```python
from build123d import *

# Parameters (mm, degrees)
CROQUIS1_R                   = 6
SALIENTE_EXTRUIR1_DEPTH      = 16.5
CROQUIS2_R                   = 4.2
CORTAR_EXTRUIR1_DEPTH        = 14.5
CROQUIS3_R                   = 2.6
SALIENTE_EXTRUIR2_DEPTH      = 6
CORTAR_EXTRUIR4_START        = -6
CORTAR_EXTRUIR4_DEPTH        = 6
CORTAR_EXTRUIR5_START        = -6
CORTAR_EXTRUIR5_DEPTH        = 6
SALIENTE_EXTRUIR3_DEPTH      = 6
SALIENTE_EXTRUIR3_DEPTH_BACK = 12
CROQUIS13_R                  = 7
CROQUIS13_R_2                = 4.7
CORTAR_EXTRUIR9_REACH        = 26.581
CORTAR_EXTRUIR9_END_RADIUS   = 7
CROQUIS14_R                  = 1.4


with BuildPart() as part:
    # Croquis1 → Saliente-Extruir1 (new body)
    with BuildSketch(Plane(origin=(0, 0, 0), x_dir=(1, 0, 0), z_dir=(0, 1, 0))):
        with Locations(Location((0, 0, 0), (0, 0, 270))):
            Circle(CROQUIS1_R)
    extrude(amount=SALIENTE_EXTRUIR1_DEPTH)

    # Croquis2 → Cortar-Extruir1 (cut)
    with BuildSketch(Plane.XZ):
        with Locations(Location((0, 0, 0), (0, 0, 270))):
            Circle(CROQUIS2_R)
    extrude(amount=-CORTAR_EXTRUIR1_DEPTH, mode=Mode.SUBTRACT)

    # Croquis3 → Saliente-Extruir2 (add)
    with BuildSketch(Plane(origin=(0, 16.5, 0), x_dir=(1, 0, 0), z_dir=(0, 1, 0))):
        with Locations(Location((0, 0, 0), (0, 0, 270))):
            Circle(CROQUIS3_R)
    extrude(amount=SALIENTE_EXTRUIR2_DEPTH)

    # Croquis7 → Cortar-Extruir4 (cut)
    with BuildSketch(Plane(origin=(0, 22.5, 0), x_dir=(1, 0, 0), z_dir=(0, 1, 0)).offset(CORTAR_EXTRUIR4_START)):
        with BuildLine():
            Line((-1.774823935, -1.9), (1.774823935, -1.9))
            ThreePointArc((1.774823935, -1.9), (0, -2.6), (-1.774823935, -1.9))
        make_face()
        with BuildLine():
            Line((-1.774823935, 1.9), (1.774823935, 1.9))
            ThreePointArc((1.774823935, 1.9), (0, 2.6), (-1.774823935, 1.9))
        make_face()
    extrude(amount=CORTAR_EXTRUIR4_DEPTH, mode=Mode.SUBTRACT)

    # Croquis10 → Cortar-Extruir5 (cut)
    with BuildSketch(Plane(origin=(0, 22.5, 0), x_dir=(1, 0, 0), z_dir=(0, 1, 0)).offset(CORTAR_EXTRUIR5_START)):
        with BuildLine():
            Line((-1.8, 0.7), (-2.503996805, 0.7))
            ThreePointArc((-2.503996805, 0.7), (-2.6, 0), (-2.503996805, -0.7))
            Line((-2.503996805, -0.7), (-1.8, -0.7))
            Line((-1.8, -0.7), (-1.8, 0.7))
        make_face()
        with BuildLine():
            Line((2.503996805, 0.7), (1.8, 0.7))
            Line((1.8, 0.7), (1.8, -0.7))
            Line((1.8, -0.7), (2.503996805, -0.7))
            ThreePointArc((2.503996805, -0.7), (2.6, 0), (2.503996805, 0.7))
        make_face()
    extrude(amount=CORTAR_EXTRUIR5_DEPTH, mode=Mode.SUBTRACT)

    # Croquis13 → Saliente-Extruir3 (add, two sides: drawn at the far end of the back side and taken through both)
    with BuildSketch(Plane(origin=(0, 16.5, 0), x_dir=(1, 0, 0), z_dir=(0, 1, 0)).offset(-SALIENTE_EXTRUIR3_DEPTH_BACK)):
        with Locations(Location((0, 0, 0), (0, 0, 270))):
            Circle(CROQUIS13_R)
        with Locations(Location((0, 0, 0), (0, 0, 270))):
            Circle(CROQUIS13_R_2, mode=Mode.SUBTRACT)
    extrude(amount=SALIENTE_EXTRUIR3_DEPTH + SALIENTE_EXTRUIR3_DEPTH_BACK)

    # Cortar-Extruir9: up to this cylinder (the profile starts inside it)
    cortar_extruir9_end = Plane(origin=(0, 10, 0), z_dir=(0, 1, 0)) * Cylinder(CORTAR_EXTRUIR9_END_RADIUS, 68.162, mode=Mode.PRIVATE)
    # Croquis14 → Cortar-Extruir9 (cut, up to the surface)
    with BuildSketch(Plane.XY, mode=Mode.PRIVATE) as cortar_extruir9_sk1:
        with Locations((0, 10)):
            Circle(CROQUIS14_R)
    cortar_extruir9_tool1 = extrude(cortar_extruir9_sk1.sketch, amount=-CORTAR_EXTRUIR9_REACH, mode=Mode.PRIVATE) & cortar_extruir9_end
    add(cortar_extruir9_tool1.solids().sort_by_distance((0, 10, 0))[0], mode=Mode.SUBTRACT)


solid = part.part
```
Verification items for the finished model (mm, model axes). A direction names the side the tool comes from. Give positions to 0.01 mm unless a question says otherwise; leave off trailing zeros. Order: outer loops, then holes, each group sorted by start corner. A loop starts at its lowest first (then second) coordinate and runs counter-clockwise, first axis right, second up. Notation, with made-up numbers: (0.5, 59) -> (40.5, 59) arc R18 ccw to (40.5, 63) -> close; hole circle Ø5 at (49, -33.75). An arc over 180 degrees is marked (long way). Use a Markdown table: item, result.
1) Section check C-C, the plane z = 0. Record the boundary of the cut face in (x, y).
Results:
| item | result |
|---|---|
| outline | (-7, 4.5) -> (-6, 4.5) -> (-6, 0) -> (-4.2, 0) -> (-4.2, 14.5) -> (4.2, 14.5) -> (4.2, 0) -> (6, 0) -> (6, 4.5) -> (7, 4.5) -> (7, 22.5) -> (4.7, 22.5) -> (4.7, 16.5) -> (1.8, 16.5) -> (1.8, 22.5) -> (-1.8, 22.5) -> (-1.8, 16.5) -> (-4.7, 16.5) -> (-4.7, 22.5) -> (-7, 22.5) -> close |
2) Mould release check, pull along X, two halves, no side actions. Record for faces 1 (the cylindrical face through (1.802, 2.218, 5.723)), 2 (the flat face through (-5, 22.5, 1)), 3 (the flat face through (-2, 16.5, 0)): pulls with the +X half, pulls with the -X half, needs draft (parallel to the pull), parting line crosses it, or undercut.
Results:
| item | result |
|---|---|
| face 1 | parting line crosses it |
| face 2 | needs draft |
| face 3 | undercut |
3) Section check B-B, the plane z = -5.5. Record the boundary of the cut face in (x, y), then the cut area to 3 significant figures.
Results:
| item | result |
|---|---|
| outline | (-4.33, 4.5) -> (-2.4, 4.5) -> (-2.4, 0) -> (2.4, 0) -> (2.4, 4.5) -> (4.33, 4.5) -> (4.33, 22.5) -> (-4.33, 22.5) -> close; hole circle Ø2.8 at (0, 10) |
| area | 171 mm² |
4) Section check D-D, the plane y = 10. Record the boundary of the cut face in (x, z), then the cut area to 3 significant figures.
Results:
| item | result |
|---|---|
| outline | (-1.4, -6.86) -> (-1.4, -3.96) arc R4.2 cw (long way) to (1.4, -3.96) -> (1.4, -6.86) arc R7 ccw (long way) to start |
| area | 90.6 mm² |
5) Tool access check on faces 4 (the flat face through (0, 22.5, 0)), 5 (the cylindrical face through (-1.4, 10.06, -5.46)), 6 (the cylindrical face through (-2.23, 19.46, 1.34)), 7 (the flat face through (0, 14.5, 0)). Record the directions out of +Z, -Z, +X, -X, +Y, -Y that give a thin tool (end or side, any length) a straight path to the whole face; none if there is none.
Results:
| item | result |
|---|---|
| face 4 | +Z, -Z, +X, -X, +Y |
| face 5 | -Z |
| face 6 | +Y |
| face 7 | -Y |
6) Material ranges on probe 1 along X at (y, z) = (19.2, 0); probe 2 along Z at (x, y) = (0, 18.3); probe 3 along X at (y, z) = (5.5, 0), recorded low to high.
Results:
| item | result |
|---|---|
| probe 1 | -7 to -4.7, -1.8 to 1.8, 4.7 to 7 |
| probe 2 | -7 to -4.7, -1.9 to 1.9, 4.7 to 7 |
| probe 3 | -7 to -4.2, 4.2 to 7 |
7) Section check A-A, the plane x = 0. Record the boundary of the cut face in (y, z), then the cut area to 3 significant figures.
Results:
| item | result |
|---|---|
| outline | (0, -6) -> (4.5, -6) -> (4.5, -7) -> (8.6, -7) -> (8.6, -4.2) -> (0, -4.2) -> close; (0, 4.2) -> (14.5, 4.2) -> (14.5, -4.2) -> (11.4, -4.2) -> (11.4, -7) -> (22.5, -7) -> (22.5, -4.7) -> (16.5, -4.7) -> (16.5, -1.9) -> (22.5, -1.9) -> (22.5, 1.9) -> (16.5, 1.9) -> (16.5, 4.7) -> (22.5, 4.7) -> (22.5, 7) -> (4.5, 7) -> (4.5, 6) -> (0, 6) -> close |
| area | 143 mm² |
8) Depth check by flat-ended pin: pin 1 Ø2.5 at (x, y) = (0, 10) entering from -Z; pin 2 Ø0.6 at (x, y) = (2, 20) entering from -Z; pin 3 Ø8 at (x, y) = (4.5, 7.5) entering from -Z. Enter the tip coordinate at first touch or a pass-through.
Results:
| item | result |
|---|---|
| pin 1 | z = 4.01 |
| pin 2 | z = -6.79 |
| pin 3 | z = -6.98 |
